Can you work these out from the model? Positions are in its coordinate system, mm. Give positions to 0.01 mm unless a question says otherwise; leave off trailing zeros. Order: outer loops, then holes, each group sorted by start corner. A loop starts at its lowest first (then second) coordinate and runs counter-clockwise, first axis right, second up. Notation, with made-up numbers: (0, -5) - (4, -5) arc R21 cw to (4, 22) - close; hole circle Ø10 at (71, -10.5). An arc over 180 degrees is marked (long way). Use one line per item in the form item = value. Start each with the question number.
1) Suppose I cut it at C-C, the plane z = 0.3. Write out the boundary of the cut face in (x, y), and give its area (3 significant figures).
2) Suppose I cut it at B-B, the plane x = 12.7. Write out the boundary of the cut face in (y, z).
3) Suppose I cut it at A-A, the plane y = -19.05. Write out the boundary of the cut face in (x, z).
4) Please list where these lines run through material, in increasing order: probe 1 along Y at (x, z) = (-12.7, -1.25); probe 2 along Y at (x, z) = (-13, 0.2); probe 3 along X at (y, z) = (26, 0.7).
5) We'd pull the mould along X, two halves only. Please class faces 1 (the flat face through (0, -31.75, 0)), 2 (the flat face through (25.4, -8, 0)), 3 (the cylindrical face through (10.294, -16.844, -0.033)), 4 (the cylindrical face through (5.462, 9.012, -0.033)): released by +X, released by -X, zero draft, split by the parting line, or undercut.
6) For pin 1 (5 mm diameter, centred on x = -13.94, y = 23.7, fed in from -Z); pin 2 (1.5 mm diameter, centred on x = 16.5, z = -1, fed in from +Y), each with a flat end and sliding along its axis, tell me the tip position at first contact or that it passes through.
7) Suppose I cut it at D-D, the plane x = -12.7. Write out the boundary of the cut face in (y, z), and give its area (3 significant figures).
```python
from build123d import *

# Parameters (mm, degrees)
BOSS_EXTRUDE1_DEPTH      = 2.3876
BOSS_EXTRUDE1_DEPTH_BACK = 2.3876
SKETCH3_R                = 3.2639


with BuildPart() as part:
    # Sketch3 → Boss-Extrude1 (new, two sides: drawn at the far end of the back side and taken through both)
    with BuildSketch(Plane.XY.offset(-BOSS_EXTRUDE1_DEPTH_BACK)):
        Polygon((25.4, -31.75), (25.4, 15.6464), (-2.4892, 31.75), (-25.4, 31.75), (-25.4, -31.75), align=None)
        with Locations((12.7, -19.05)):
            Circle(SKETCH3_R, mode=Mode.SUBTRACT)
        with Locations((8.052122612, 10.9982)):
            Circle(SKETCH3_R, mode=Mode.SUBTRACT)
        with Locations((-12.7, -19.05)):
            Circle(SKETCH3_R, mode=Mode.SUBTRACT)
        with Locations((-13.944922644, 23.6982)):
            Circle(SKETCH3_R, mode=Mode.SUBTRACT)
    extrude(amount=BOSS_EXTRUDE1_DEPTH + BOSS_EXTRUDE1_DEPTH_BACK)


solid = part.part
```
Result sheet:
q1.outline = (-25.4, -31.75) - (25.4, -31.75) - (25.4, 15.65) - (-2.49, 31.75) - (-25.4, 31.75) - close; hole circle Ø6.53 at (-13.94, 23.7); hole circle Ø6.53 at (-12.7, -19.05); hole circle Ø6.53 at (8.05, 11); hole circle Ø6.53 at (12.7, -19.05)
q1.area = 2,870 mm²
q2.outline = (-31.75, -2.39) - (-22.31, -2.39) - (-22.31, 2.39) - (-31.75, 2.39) - close; (-15.79, -2.39) - (22.98, -2.39) - (22.98, 2.39) - (-15.79, 2.39) - close
q3.outline = (-25.4, -2.39) - (-15.96, -2.39) - (-15.96, 2.39) - (-25.4, 2.39) - close; (-9.44, -2.39) - (9.44, -2.39) - (9.44, 2.39) - (-9.44, 2.39) - close; (15.96, -2.39) - (25.4, -2.39) - (25.4, 2.39) - (15.96, 2.39) - close
q4.probe_1 = -31.75 to -22.31, -15.79 to 20.68, 26.72 to 31.75
q4.probe_2 = -31.75 to -22.3, -15.8 to 20.57, 26.82 to 31.75
q4.probe_3 = -25.4 to -16.26, -11.63 to 7.47
q5.face_1 = zero draft
q5.face_2 = released by +X
q5.face_3 = undercut
q5.face_4 = undercut
q6.pin_1 = through
q6.pin_2 = 21.22
q7.outline = (-31.75, -2.39) - (-22.31, -2.39) - (-22.31, 2.39) - (-31.75, 2.39) - close; (-15.79, -2.39) - (20.68, -2.39) - (20.68, 2.39) - (-15.79, 2.39) - close; (26.72, -2.39) - (31.75, -2.39) - (31.75, 2.39) - (26.72, 2.39) - close
q7.area = 243 mm²
